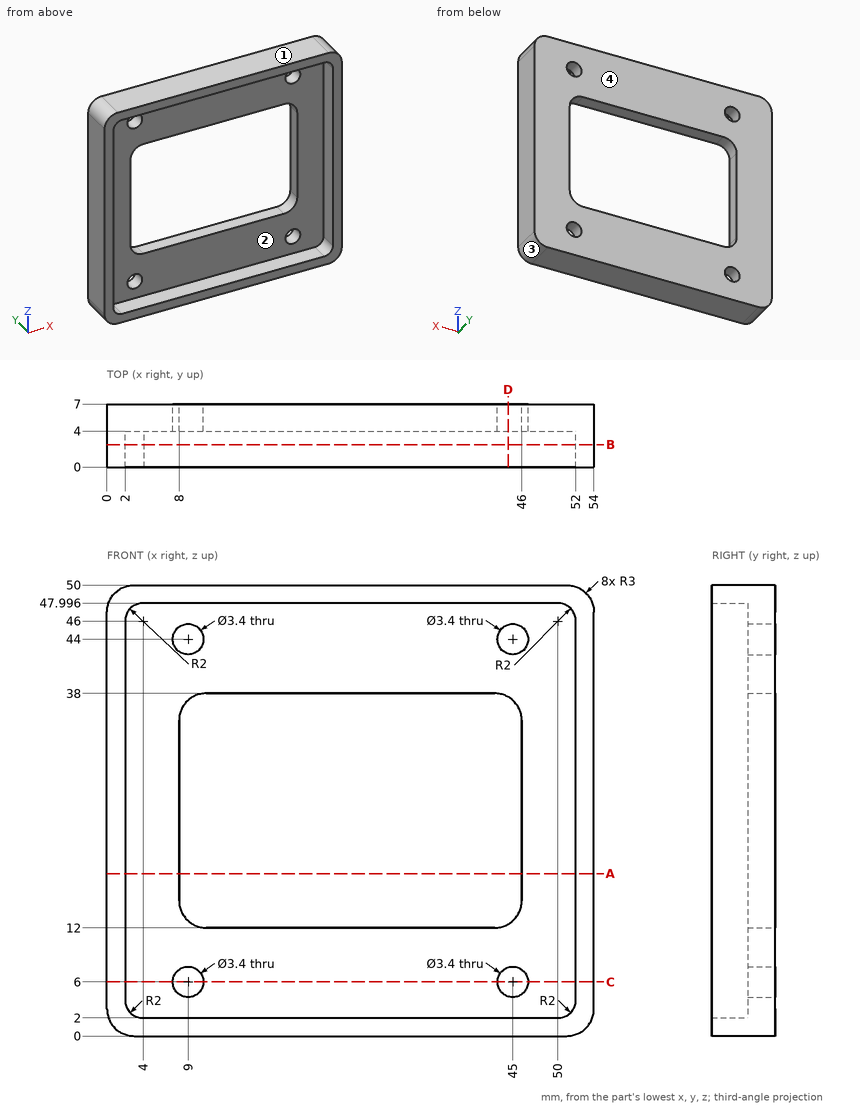
Part print with two shaded views. Sizes in mm from the minimum x, y, z corner. Give positions to 0.01 mm unless a question says otherwise; leave off trailing zeros. Order: outer loops, then holes, each group sorted by start corner. A loop starts at its lowest first (then second) coordinate and runs counter-clockwise, first axis right, second up. Notation, with made-up numbers: (-3, 35) - (9, 35) arc R17 cw to (9, 50) - close; hole circle Ø2 at (-30.75, 81.25). An arc over 180 degrees is marked (long way). Write each question's results on one line, items separated by ' | '.
1. Saw through at D-D on x = 44.5. List the corners of the cut face in (y, z) (1 decimal).
Calculated:
outline: (0, 0) - (7, 0) - (7, 4.4) - (4, 4.4) - (4, 2) - (0, 2) - close; (0, 48) - (4, 48) - (4, 45.6) - (7, 45.6) - (7, 50) - (0, 50) - close; (4, 7.6) - (7, 7.6) - (7, 12.4) - (4, 12.4) - close; (4, 37.6) - (7, 37.6) - (7, 42.4) - (4, 42.4) - close
2. Pull direction Z, two halves, no side cores. Call the marked faces 1, 2, 3 and 4: released by +Z, released by -Z, zero draft, split by the parting line, or undercut.
Calculated:
face 1: released by +Z | face 2: undercut | face 3: released by -Z | face 4: zero draft
3. Pin check, flat tip, straight feed: pin 1 (4.5 mm diameter, centred on x = 9, z = 44, fed in from -Y). Stop position of the tip, or through.
Calculated:
pin 1: stops at y = 4
4. Saw through at A-A on z = 18. List the corners of the cut face in (x, y).
Calculated:
outline: (0, 0) - (2, 0) - (2, 4) - (8, 4) - (8, 7) - (0, 7) - close; (46, 4) - (52, 4) - (52, 0) - (54, 0) - (54, 7) - (46, 7) - close
5. Probe L1, parallel to Z at x = 41, y = 6; L2, parallel to X at y = 5, z = 25; L3, parallel to Z at x = 9, y = 6.2 (1 decimal). List the from-to ranges inside material, lowest first. Write a range as from..to.
Calculated:
L1: z = 0..12, 38..50 | L2: x = 0..8, 46..54 | L3: z = 0..4.3, 7.7..12.8, 37.2..42.3, 45.7..50
6. Saw through at C-C on z = 6. List the corners of the cut face in (x, y).
Calculated:
outline: (0, 0) - (2, 0) - (2, 4) - (7.3, 4) - (7.3, 7) - (0, 7) - close; (10.7, 4) - (43.3, 4) - (43.3, 7) - (10.7, 7) - close; (46.7, 4) - (52, 4) - (52, 0) - (54, 0) - (54, 7) - (46.7, 7) - close
7. Saw through at B-B on y = 2.5. List the corners of the cut face in (x, z).
Calculated:
outline: (0, 3) arc R3 ccw to (3, 0) - (51, 0) arc R3 ccw to (54, 3) - (54, 47) arc R3 ccw to (51, 50) - (3, 50) arc R3 ccw to (0, 47) - close; hole (2, 4) arc R2 ccw to (4, 2) - (50, 2) arc R2 ccw to (52, 4) - (52, 46) arc R2 ccw to (50, 48) - (4.12, 48) arc R2 ccw to (2, 46) - close
